```python
from build123d import *

# Parameters (mm, degrees)
BOSS_EXTRUDE1_DEPTH = 2.032
CUT_EXTRUDE2_DEPTH  = 24.892
FILLET1_R           = 15.24
CUT_EXTRUDE3_DEPTH  = 27.869973793


with BuildPart() as part:
    # Sketch1 → Boss-Extrude1 (new body)
    with BuildSketch(Plane.XY):
        with BuildLine():
            Line((0, 0), (15.748, 0))
            Line((15.748, 0), (18.796, 3.5687))
            Line((18.796, 3.5687), (15.748, 7.1374))
            Line((15.748, 7.1374), (1.249093629, 7.1374))
            ThreePointArc((1.249093629, 7.1374), (1.020493629, 7.076146815), (0.853146815, 6.9088))
            ThreePointArc((0.853146815, 6.9088), (0.338867933, 6.695778712), (0, 7.1374))
            Line((0, 7.1374), (0, 8.382))
            ThreePointArc((0, 8.382), (-0.671156766, 9.42306338), (-1.896435629, 9.241525307))
            ThreePointArc((-1.896435629, 9.241525307), (-3.167624386, 8.846252494), (-4.312815757, 9.525))
            ThreePointArc((-4.312815757, 9.525), (-22.986492034, 3.466471629), (-4.196095201, -2.219734364))
            ThreePointArc((-4.196095201, -2.219734364), (-2.373522466, -0.589120746), (0, 0))
        make_face()
        with BuildLine():
            Line((-14.732, 9.9187), (-14.732, -2.7813))
            ThreePointArc((-14.732, -2.7813), (-21.082, 3.5687), (-14.732, 9.9187))
        make_face(mode=Mode.SUBTRACT)
    extrude(amount=BOSS_EXTRUDE1_DEPTH)

    # Sketch2 → Cut-Extrude2 (cut)
    with BuildSketch(Plane(origin=(18.796, 0, 0), x_dir=(0, 0, -1), z_dir=(1, 0, 0))):
        Polygon((0, 0.9144), (-1.3589, 0.9144), (-1.3589, 2.1844), (0, 2.968961281), align=None)
        Polygon((-0.762, 3.7973), (-2.032, 3.064065158), (-2.032, 7.9883), (-0.762, 7.9883), align=None)
    extrude(amount=-CUT_EXTRUDE2_DEPTH, mode=Mode.SUBTRACT)

    # Fillet1
    # the kernel refuses this fillet: 15.24 mm, written as the material it adds along each edge
    with BuildSketch(Plane(origin=(-6.096, 0.9144, 1.3589), x_dir=(0, 0, -1), z_dir=(0, 1, 0))) as fillet1_piece_1_section:
        with BuildLine():
            CenterArc((15.24, -6.29068063), FILLET1_R, 155.620767223, 24.379232777)
            Line((0, -6.29068063), (-0.3048, -6.29068063))
            Line((-0.3048, -6.29068063), (-0.3048, 0))
            Line((-0.3048, 0), (0, 0.3048))
            ThreePointArc((0, 0.3048), (0.67945, 0.3048), (1.081278, 0.125813613))
            Line((1.081278, 0.125813613), (1.3589, 0))
        make_face()
    fillet1_piece_1 = extrude(amount=16.996701575, mode=Mode.PRIVATE)
    fillet1_piece_1 = split(fillet1_piece_1, bisect_by=Plane(origin=(-4.21750285, 2.15532175, 1.409265006), z_dir=(0, -0.8660254037844416, -0.49999999999999506)), keep=Keep.TOP, mode=Mode.PRIVATE)
    add(fillet1_piece_1)
    with BuildSketch(Plane(origin=(-6.096, 7.9883, 0.762), x_dir=(0, 0, 1), z_dir=(0, -1, 0))) as fillet1_piece_2_section:
        with BuildLine():
            CenterArc((15.24, -6.090706035), FILLET1_R, 156.443535691, 23.556464309)
            Line((0, -6.090706035), (-0.3048, -6.090706035))
            Line((-0.3048, -6.090706035), (-0.3048, 0))
            Line((-0.3048, 0), (0, 0.3048))
            ThreePointArc((0, 0.3048), (0.635, 0.3048), (0.9906, 0.121814121))
            Line((0.9906, 0.121814121), (1.27, 0))
        make_face()
    fillet1_piece_2 = extrude(amount=19.417765087, mode=Mode.PRIVATE)
    fillet1_piece_2 = split(fillet1_piece_2, bisect_by=Plane(origin=(-4.154309829, 4.225398766, 0.020511187), z_dir=(0, 0.8660254037844416, 0.49999999999999506)), keep=Keep.TOP, mode=Mode.PRIVATE)
    add(fillet1_piece_2)

    # Sketch3 → Cut-Extrude3 (cut, through all)
    with BuildSketch(Plane.XY.offset(0.762)):
        Polygon((18.796, 7.9883), (18.796, 3.5687), (16.25112476, 6.54832476), (15.0368, 5.334), (13.5128, 5.334), (12.09675, 6.75005), (11.8618, 6.5151), (10.3378, 6.5151), (10.10285, 6.75005), (8.6868, 5.334), (7.1628, 5.334), (6.731, 5.7658), (5.5118, 4.5466), (3.9878, 4.5466), (0.5461, 7.9883), align=None)
    extrude(amount=-CUT_EXTRUDE3_DEPTH, mode=Mode.SUBTRACT)


solid = part.part
```
Design review of the part built by this model. Coordinates are the model's own, in mm. A direction names the side the tool comes from. Round coordinates to 2 decimals unless told otherwise and drop trailing zeros. Write each loop counter-clockwise with the first axis right and the second up, starting at its lowest first coordinate (ties: lowest second). Pieces come first, ordered by that corner, then holes. Notation, with made-up numbers: (18, 46) -> (45, 46) arc R28 cw to (45, 67) -> close; hole circle Ø4 at (-2, 57.5). An arc over 180 degrees is marked (long way). Write item = value, one per line. Start each with the question number.
1) Wall thickness on probe 1 along Y at (x, z) = (4.5, 0.95); probe 2 along X at (y, z) = (4.75, 0.7); probe 3 along Z at (x, y) = (7.5, 1): over which ranges is each line inside the solid? List them lowest first. Write a range as from..to.
2) Take a section at A-A, the plane x = 11. State the section outline as (y, z) points, plus the area to 3 significant figures.
3) Tool access review of faces 4 (the face through (-3.2, 5.6, 1.1)), 5 (the face through (-21.08, 3.43, 1)), 6 (the face through (9.4, 6.05, 0.39)), 7 (the face through (0, 7.9, 0.6)): name each direction out of +Z, -Z, +X, -X, +Y, -Y from which nothing blocks a thin tool from reaching the whole face with its end or side.
4) Clearance check with flat-ended pins moving along their axes: pin 1 (4.5 mm diameter, centred on x = 7.5, y = 5.5, fed in from +Z); pin 2 (1 mm diameter, centred on y = -4.5, z = 0.5, fed in from -X); pin 3 (0.6 mm diameter, centred on x = 8, z = 0.5, fed in from +Y). State where each tip first meets the part, or that it passes through.
5) Mouldability with a two-part tool opening along Y and no side actions: class faces 1 (the face through (-2.404, -0.605, 1.002)), 2 (the face through (-2.3, 7.988, 1.5)), 3 (the face through (12.815, 6.032, 0.386)) as +Y half, -Y half, draft (parallel to the pull), parting line (faces both ways), or undercut.
6) Take a section at D-D, the plane y = -4.75. State the section outline as (x, z) points.
7) Take a section at B-B, the plane y = -1.25. State the section outline as (x, z) points.
Results list:
q1.probe_1 = 0..0.91, 2.42..3.69
q1.probe_2 = -22.92..-20.97, -14.73..3.78, 5.72..17.79
q1.probe_3 = 1.36..2.03
q2.outline = (0, 0) -> (0.91, 0) -> (0.91, 1.36) -> (2.18, 1.36) -> (2.97, 0) -> (6.52, 0) -> (6.52, 0.76) -> (3.8, 0.76) -> (3.06, 2.03) -> (0, 2.03) -> close
q2.area = 7.06 mm²
q3.face_4 = +Z, +X
q3.face_5 = +Z, -Z
q3.face_6 = +Z, -Z, +Y
q3.face_7 = +Z, -Z, +X, +Y
q4.pin_1 = 1.71
q4.pin_2 = -19.67
q4.pin_3 = 5.33
q5.face_1 = -Y half
q5.face_2 = undercut
q5.face_3 = +Y half
q6.outline = (-18.75, 0) -> (-6.65, 0) -> (-6.65, 2.03) -> (-18.75, 2.03) -> close
q7.outline = (-21.79, 0) -> (-18.87, 0) -> (-18.87, 2.03) -> (-21.79, 2.03) -> close; (-14.73, 0) -> (-3.34, 0) -> (-3.34, 2.03) -> (-14.73, 2.03) -> close
